```python
from build123d import *

# Parameters (mm, degrees)
BOSS_EXTRUDE1_DEPTH = 50
BOSS_EXTRUDE2_START = 50
SKETCH2_3_R         = 23
BOSS_EXTRUDE2_DEPTH = 127.5
BOSS_EXTRUDE3_DEPTH = 177.5
SKETCH3_W           = 52.5
SKETCH3_H           = 52.5
BOSS_EXTRUDE4_DEPTH = 70
SKETCH4_W           = 150
SKETCH4_H           = 50
BOSS_EXTRUDE5_DEPTH = 2.5
SKETCH4_4_W         = 155
SKETCH4_4_H         = 55
SKETCH4_4_W_2       = 150
SKETCH4_4_H_2       = 50
BOSS_EXTRUDE6_DEPTH = 55
SKETCH5_W           = 47.5
SKETCH5_H           = 47.5
CUT_EXTRUDE4_DEPTH  = 50
SKETCH6_W           = 20
SKETCH6_H           = 20
CUT_EXTRUDE5_DEPTH  = 20
SKETCH7_W           = 7.5
SKETCH7_H           = 52.5
SKETCH7_R           = 1.65
BOSS_EXTRUDE7_DEPTH = 2.5


with BuildPart() as part:
    # Sketch2 → Boss-Extrude1 (new body)
    with BuildSketch(Plane(origin=(0, 0, 0), x_dir=(1, 0, 0), z_dir=(0, 1, 0))):
        with BuildLine():
            ThreePointArc((-26.25, -11.459990061), (-20.253319138, -20.253319138), (-11.459990061, -26.25))
            Line((-11.459990061, -26.25), (11.459990061, -26.25))
            ThreePointArc((11.459990061, -26.25), (20.253319138, -20.253319138), (26.25, -11.459990061))
            Line((26.25, -11.459990061), (26.25, 11.459990061))
            ThreePointArc((26.25, 11.459990061), (20.253319138, 20.253319138), (11.459990061, 26.25))
            Line((11.459990061, 26.25), (-11.459990061, 26.25))
            ThreePointArc((-11.459990061, 26.25), (-20.253319138, 20.253319138), (-26.25, 11.459990061))
            Line((-26.25, 11.459990061), (-26.25, -11.459990061))
        make_face()
        Polygon((-7.1, 17.237560734), (7.1, 17.237560734), (11.378165495, 14.767560734), (18.478165495, 2.47), (18.478165495, -2.47), (11.378165495, -14.767560734), (7.1, -17.237560734), (-7.1, -17.237560734), (-11.378165495, -14.767560734), (-18.478165495, -2.47), (-18.478165495, 2.47), (-11.378165495, 14.767560734), align=None, mode=Mode.SUBTRACT)
    extrude(amount=BOSS_EXTRUDE1_DEPTH)

    # Sketch2<3> → Boss-Extrude2 (add)
    with BuildSketch(Plane(origin=(0, 0, 0), x_dir=(1, 0, 0), z_dir=(0, 1, 0)).offset(BOSS_EXTRUDE2_START)):
        with BuildLine():
            ThreePointArc((-26.25, -11.459990061), (-20.253319138, -20.253319138), (-11.459990061, -26.25))
            Line((-11.459990061, -26.25), (11.459990061, -26.25))
            ThreePointArc((11.459990061, -26.25), (20.253319138, -20.253319138), (26.25, -11.459990061))
            Line((26.25, -11.459990061), (26.25, 11.459990061))
            ThreePointArc((26.25, 11.459990061), (20.253319138, 20.253319138), (11.459990061, 26.25))
            Line((11.459990061, 26.25), (-11.459990061, 26.25))
            ThreePointArc((-11.459990061, 26.25), (-20.253319138, 20.253319138), (-26.25, 11.459990061))
            Line((-26.25, 11.459990061), (-26.25, -11.459990061))
        make_face()
        with Locations(Location((0, 0, 0), (0, 0, 270))):
            Circle(SKETCH2_3_R, mode=Mode.SUBTRACT)
    extrude(amount=BOSS_EXTRUDE2_DEPTH)

    # Sketch2<4> → Boss-Extrude3 (add)
    with BuildSketch(Plane(origin=(0, 0, 0), x_dir=(1, 0, 0), z_dir=(0, 1, 0))):
        with BuildLine():
            Line((-26.25, 26.25), (-26.25, 11.459990061))
            ThreePointArc((-26.25, 11.459990061), (-20.253319138, 20.253319138), (-11.459990061, 26.25))
            Line((-11.459990061, 26.25), (-26.25, 26.25))
        make_face()
        with BuildLine():
            ThreePointArc((11.459990061, 26.25), (20.253319138, 20.253319138), (26.25, 11.459990061))
            Line((26.25, 11.459990061), (26.25, 26.25))
            Line((26.25, 26.25), (11.459990061, 26.25))
        make_face()
        with BuildLine():
            ThreePointArc((26.25, -11.459990061), (20.253319138, -20.253319138), (11.459990061, -26.25))
            Line((11.459990061, -26.25), (26.25, -26.25))
            Line((26.25, -26.25), (26.25, -11.459990061))
        make_face()
        with BuildLine():
            Line((-26.25, -11.459990061), (-26.25, -26.25))
            Line((-26.25, -26.25), (-11.459990061, -26.25))
            ThreePointArc((-11.459990061, -26.25), (-20.253319138, -20.253319138), (-26.25, -11.459990061))
        make_face()
    extrude(amount=BOSS_EXTRUDE3_DEPTH)

    # Sketch3 → Boss-Extrude4 (add)
    with BuildSketch(Plane.XZ):
        Rectangle(SKETCH3_W, SKETCH3_H)
    extrude(amount=BOSS_EXTRUDE4_DEPTH)



with BuildPart() as body_2:
    # Sketch4 → Boss-Extrude5 (new body)
    with BuildSketch(Plane(origin=(0, -70, 0), x_dir=(-1, 0, 0), z_dir=(0, -1, 0))):
        with Locations((0, -53.75)):
            Rectangle(SKETCH4_W, SKETCH4_H)
    extrude(amount=-BOSS_EXTRUDE5_DEPTH)


with BuildPart() as part_1:
    add(part.part)

    add(body_2.part)  # Boss-Extrude6 merges body 2
    # Sketch4<4> → Boss-Extrude6 (add)
    with BuildSketch(Plane(origin=(0, -70, 0), x_dir=(-1, 0, 0), z_dir=(0, -1, 0))):
        with Locations((0, -53.75)):
            Rectangle(SKETCH4_4_W, SKETCH4_4_H)
        with Locations((0, -53.75)):
            Rectangle(SKETCH4_4_W_2, SKETCH4_4_H_2, mode=Mode.SUBTRACT)
    extrude(amount=-BOSS_EXTRUDE6_DEPTH)

    # Sketch5 → Cut-Extrude4 (cut)
    with BuildSketch(Plane.XZ.offset(70)):
        Rectangle(SKETCH5_W, SKETCH5_H)
    extrude(amount=-CUT_EXTRUDE4_DEPTH, mode=Mode.SUBTRACT)

    # Sketch6 → Cut-Extrude5 (cut)
    with BuildSketch(Plane.XY.offset(26.25)):
        with Locations((0, 10)):
            Rectangle(SKETCH6_W, SKETCH6_H)
    extrude(amount=-CUT_EXTRUDE5_DEPTH, mode=Mode.SUBTRACT)

    # Sketch7 → Boss-Extrude7 (add)
    # profile 1 of 2: a face of its own
    with BuildSketch(Plane.XZ.offset(70)):
        with Locations((-30, 0)):
            Rectangle(SKETCH7_W, SKETCH7_H)
        with Locations(Location((-30, 0, 0), (0, 0, 270))):
            Circle(SKETCH7_R, mode=Mode.SUBTRACT)
    # profile 2 of 2: a face of its own
    with BuildSketch(Plane.XZ.offset(70)):
        with Locations((30, 0)):
            Rectangle(SKETCH7_W, SKETCH7_H)
        with Locations(Location((30, 0, 0), (0, 0, 270))):
            Circle(SKETCH7_R, mode=Mode.SUBTRACT)
    extrude(amount=-BOSS_EXTRUDE7_DEPTH)


solid = part_1.part
```
The model under review builds one solid part; all positions refer to its coordinate system, in mm. A direction names the side the tool comes from. Give positions to 0.01 mm unless a question says otherwise; leave off trailing zeros. Write each loop counter-clockwise with the first axis right and the second up, starting at its lowest first coordinate (ties: lowest second). Pieces come first, ordered by that corner, then holes. Notation, with made-up numbers: M -10,-16.5 L 38,-16.5 A16 cw 38,9.5 Z; hole C 50.25,-40 d3. An arc over 180 degrees is marked long. Write each question's results on one line, items separated by ' | '. Start each with the question number.
1. Mouldability with a two-part tool opening along Y and no side actions: class faces 1 (the flat face through (-10, 10, 21)), 2 (the flat face through (-52, -43, 26.25)), 3 (the flat face through (0, -15, 27)) as released by +Y, released by -Y, zero draft, split by the parting line, or undercut.
2. For faces 4 (the flat face through (10, 10, 21)), 5 (the flat face through (0, -20, 0)), 6 (the flat face through (14.88, 24.65, -8.7)), 7 (the flat face through (-26.25, 57, 0)), 8 (the flat face through (-1, -70, 52)), list the 3-axis set-ups (+Z, -Z, +X, -X, +Y, -Y) from which the entire face can be reached by the end or side of a thin tool; tool diameter is ignored.
3. We need section C-C (z = 43.5). Write out the cut boundary in (x, y), and give its area (3 significant figures).
4. We need section A-A (x = 0). Write out the cut boundary in (y, z), and give its area (3 significant figures).
5. We need section D-D (x = -45). Write out the cut boundary in (y, z).
6. We need section B-B (y = 58). Write out the cut boundary in (x, z).
7. Insertion check: pin 1 Ø7 at (x, y) = (-2.5, 29) entering from +Z; pin 2 Ø6 at (x, z) = (-15.5, 63.5) entering from +Y; pin 3 Ø8.5 at (y, z) = (13.5, 20.5) entering from -X; pin 4 Ø8.5 at (x, z) = (-2.5, 21.5) entering from -Y. Each pin has a flat end and moves straight along its axis. Give the tip position at first contact, or say it passes through.
8. For probe 1 along X at (y, z) = (-68, 0); probe 2 along X at (y, z) = (-50.5, 33); probe 3 along X at (y, z) = (-44, -2), list the stretches that pass through material, from the lowest coordinate up. Write a range as [from, to].
Results found:
1) face 1: undercut | face 2: zero draft | face 3: released by +Y
2) face 4: +Z | face 5: -Y | face 6: +Y | face 7: -Z, -X, +Y | face 8: +Z, -Z, +X, -X, -Y
3) outline: M -77.5,-70 L 77.5,-70 L 77.5,-15 L 75,-15 L 75,-67.5 L -75,-67.5 L -75,-15 L -77.5,-15 Z | area: 650 mm^2
4) outline: M -70,-26.25 L 177.5,-26.25 L 177.5,-23 L 50,-23 L 50,-17.24 L 0,-17.24 L 0,26.25 L -15,26.25 L -15,28.75 L -67.5,28.75 L -67.5,78.75 L -15,78.75 L -15,81.25 L -70,81.25 L -70,23.75 L -20,23.75 L -20,-23.75 L -70,-23.75 Z; M 20,17.24 L 50,17.24 L 50,23 L 177.5,23 L 177.5,26.25 L 20,26.25 Z | area: 3,250 mm^2
5) outline: M -70,26.25 L -15,26.25 L -15,28.75 L -67.5,28.75 L -67.5,78.75 L -15,78.75 L -15,81.25 L -70,81.25 Z
6) outline: M -26.25,-26.25 L 26.25,-26.25 L 26.25,26.25 L -26.25,26.25 Z; hole C 0,0 d46
7) pin 1: stops at z = 26.25 | pin 2: stops at y = -67.5 | pin 3: stops at x = -26.25 | pin 4: stops at y = -70
8) probe 1: x = [-33.75, -31.65], [-28.35, -23.75], [23.75, 28.35], [31.65, 33.75] | probe 2: x = [-77.5, -75], [75, 77.5] | probe 3: x = [-26.25, -23.75], [23.75, 26.25]
